Source: CAD feature listing. Evaluate the final solid. Frame: model axes, mm. A direction names the side the tool comes from. Coordinates: 2 decimals unless noted, no trailing zeros. Loops run counter-clockwise (first coordinate to the right, second up) from the corner with the lowest first, then second, coordinate; pieces in that order, holes last.
```python
from build123d import *

# Parameters (mm, degrees)
SKIZZE2_R                       = 6.25
SCHNITT_LINEAR_AUSTRAGEN1_DEPTH = 26.824842691


with BuildPart() as part:
    # Skizze1 → Rotation2 (revolve)
    with BuildSketch(Plane.XY):
        Polygon((0, 0), (0, 18), (1.1, 18), (1.1, 15), (4.35, 15), (4.35, 11.075), (0.8, 11.075), (0.8, 0), align=None)
    revolve(axis=Axis((0.8, 0, 0), (-1, 0, 0)))

    # Skizze2 → Schnitt-Linear austragen1 (cut, through all)
    with BuildSketch(Plane.ZY):
        with Locations(Location((0, 0, 0), (0, 0, 270))):
            Circle(SKIZZE2_R)
    extrude(amount=-SCHNITT_LINEAR_AUSTRAGEN1_DEPTH, mode=Mode.SUBTRACT)


solid = part.part
```
Q1. Section query D-D on z = -7.5. Return the cut outline in (x, y), then the cut area to 3 significant figures.
Q2. Section query C-C on x = 1.65. Return the cut outline in (y, z) (3 decimals).
Q3. Reachability of faces 1 (the cylindrical face through (2.55, -2.4, 10.81)), 2 (the flat face through (0, 0, 8)) from +Z, -Z, +X, -X, +Y, -Y: full face, straight path, thin tool, end or side. Return the list, or none.
Q4. Draft query along Z for faces 3 (the cylindrical face through (0.39, -5.96, 1.88)), 4 (the flat face through (4.35, -7, 9)), 5 (the cylindrical face through (0.558, -2.343, -17.847)). Return one class per face: released by +Z, released by -Z, zero draft, split by the parting line, or undercut.
Q5. First-contact query: pin 1 Ø2 at (x, z) = (2.5, -5.5) entering from +Y; pin 2 Ø1.5 at (x, y) = (3.5, 10) entering from -Z; pin 3 Ø7.5 at (y, z) = (0, 0) entering from +X; pin 4 Ø2 at (x, y) = (1.5, -5.5) entering from +Z. Flat tips, straight axial feed; report the tip coordinate or a pass-through.
Q6. Material intervals for line 1 along Z through (x, y) = (2.3, 0) (3 decimals); line 2 along Z through (x, y) = (1.45, 5), sorted ascending.
Q7. Section query A-A on z = 0. Return the cut outline in (x, y) (3 decimals).
Resolved:
1. outline: (0, -16.36) - (1.1, -16.36) - (1.1, -12.99) - (4.35, -12.99) - (4.35, -8.15) - (0.8, -8.15) - (0.8, 8.15) - (4.35, 8.15) - (4.35, 12.99) - (1.1, 12.99) - (1.1, 16.36) - (0, 16.36) - close
1. area: 62.6 mm2
2. outline: circle Ø30 at (0, 0); hole circle Ø22.15 at (0, 0)
3. face 1: +X
3. face 2: +Z, -Z, -X, +Y, -Y
4. face 3: undercut
4. face 4: zero draft
4. face 5: split by the parting line
5. pin 1: stops at y = 14.31
5. pin 2: stops at z = -11.81
5. pin 3: passes through
5. pin 4: stops at z = 17.41
6. line 1: z = -15 to -11.075, 11.075 to 15
6. line 2: z = -14.14 to -9.88, 9.88 to 14.14
7. outline: (0, -18) - (1.1, -18) - (1.1, -15) - (4.35, -15) - (4.35, -11.075) - (0.8, -11.075) - (0.8, -6.25) - (0, -6.25) - close; (0, 6.25) - (0.8, 6.25) - (0.8, 11.075) - (4.35, 11.075) - (4.35, 15) - (1.1, 15) - (1.1, 18) - (0, 18) - close
